from build123d import *

# Parameters (mm, degrees)
SKETCH1_R           = 1.054
BOSS_EXTRUDE1_DEPTH = 3
SKETCH3_R           = 1.1
BOSS_EXTRUDE2_DEPTH = 3
CUT_EXTRUDE1_DEPTH  = 23.736281859
SKETCH4_R           = 1.5
BOSS_EXTRUDE3_DEPTH = 1
FILLET1_R           = 1


with BuildPart() as part:
    # Sketch1 → Boss-Extrude1 (new body)
    with BuildSketch(Plane(origin=(0, 0, 0), x_dir=(1, 0, 0), z_dir=(0, 1, 0))):
        with BuildLine():
            Line((0, 0), (9.035898385, 0))
            ThreePointArc((9.035898385, 0), (10.767949192, 1), (10.767949192, 3))
            Line((10.767949192, 3), (1.732050808, 18.650635095))
            ThreePointArc((1.732050808, 18.650635095), (0, 19.650635095), (-1.732050808, 18.650635095))
            Line((-1.732050808, 18.650635095), (-10.767949192, 3))
            ThreePointArc((-10.767949192, 3), (-10.767949192, 1), (-9.035898385, 0))
            Line((-9.035898385, 0), (0, 0))
        make_face()
        with Locations(Location((0, 17.650635095, 0), (0, 0, 270))):
            Circle(SKETCH1_R, mode=Mode.SUBTRACT)
        with Locations(Location((-9.035898385, 2, 0), (0, 0, 270))):
            Circle(SKETCH1_R, mode=Mode.SUBTRACT)
        with Locations(Location((9.035898385, 2, 0), (0, 0, 270))):
            Circle(SKETCH1_R, mode=Mode.SUBTRACT)
    extrude(amount=BOSS_EXTRUDE1_DEPTH)

    # Sketch3 → Boss-Extrude2 (add)
    with BuildSketch(Plane(origin=(0, 3, 0), x_dir=(1, 0, 0), z_dir=(0, 1, 0))):
        with BuildLine():
            Line((-9.526279442, 14.216878365), (9.526279442, 14.216878365))
            ThreePointArc((9.526279442, 14.216878365), (10.825317547, 13.466878365), (10.825317547, 11.966878365))
            Line((10.825317547, 11.966878365), (1.299038106, -4.533121635))
            ThreePointArc((1.299038106, -4.533121635), (0, -5.283121635), (-1.299038106, -4.533121635))
            Line((-1.299038106, -4.533121635), (-10.825317547, 11.966878365))
            ThreePointArc((-10.825317547, 11.966878365), (-10.825317547, 13.466878365), (-9.526279442, 14.216878365))
        make_face()
        with Locations(Location((0, -3.783121635, 0), (0, 0, 270))):
            Circle(SKETCH3_R, mode=Mode.SUBTRACT)
        with Locations(Location((-9.526279442, 12.716878365, 0), (0, 0, 270))):
            Circle(SKETCH3_R, mode=Mode.SUBTRACT)
        with Locations(Location((9.526279442, 12.716878365, 0), (0, 0, 270))):
            Circle(SKETCH3_R, mode=Mode.SUBTRACT)
    extrude(amount=-BOSS_EXTRUDE2_DEPTH)

    # Sketch2 → Cut-Extrude1 (cut, through all)
    with BuildSketch(Plane(origin=(0, 3, 0), x_dir=(1, 0, 0), z_dir=(0, 1, 0))):
        with BuildLine():
            Line((-1, 15.918584287), (-8.035898385, 3.732050808))
            ThreePointArc((-8.035898385, 3.732050808), (-7.303847577, 3), (-7.035898385, 2))
            Line((-7.035898385, 2), (7.035898385, 2))
            ThreePointArc((7.035898385, 2), (7.303847577, 3), (8.035898385, 3.732050808))
            Line((8.035898385, 3.732050808), (1, 15.918584287))
            ThreePointArc((1, 15.918584287), (0, 15.650635095), (-1, 15.918584287))
        make_face()
    extrude(amount=-CUT_EXTRUDE1_DEPTH, mode=Mode.SUBTRACT)

    # Sketch4 → Boss-Extrude3 (add)
    with BuildSketch(Plane.XZ):
        with Locations(Location((0, 3.783121635, 0), (0, 0, 30))):
            Circle(SKETCH4_R)
        with Locations(Location((9.526279442, -12.716878365, 0), (0, 0, 270))):
            Circle(SKETCH4_R)
        with Locations(Location((-9.526279442, -12.716878365, 0), (0, 0, 270))):
            Circle(SKETCH4_R)
    extrude(amount=BOSS_EXTRUDE3_DEPTH)

    # Fillet1
    fillet1_edges = [part.edges().sort_by_distance(p)[0] for p in [
        (-1.299038106, -1, 3.033121635),
        (9.526279442, -1, -11.216878365),
        (-9.526279442, -1, -11.216878365),
    ]]
    fillet(fillet1_edges, radius=FILLET1_R - 0.0001)  # a hair under: the kernel refuses the full size


solid = part.part
Model file for the job. Use its own axes, mm. A direction names the side the tool comes from. Coordinates: 2 decimals unless noted, no trailing zeros. Order: outer loops, then holes, each group sorted by start corner. A loop starts at its lowest first (then second) coordinate and runs counter-clockwise, first axis right, second up. Notation, with made-up numbers: (69.25, -10.75) -> (76.25, -10.75) arc R16 ccw to (76.25, 13.25) -> close; hole circle Ø2 at (36, -27). An arc over 180 degrees is marked (long way). Return JSON: item names as keys, results as strings. Group by question number.
Item 1: Saw through at A-A on y = 2.2. State how many separate pieces and enclosed holes the cut face has, then the cut area to 3 significant figures.
Item 2: Pull direction X, two halves, no side cores. Call faces 1 (the flat face through (-9.5, 1.52, -9.67)), 2 (the flat face through (0, -1, 4)), 3 (the flat face through (3.03, 1.48, -16.4)), 4 (the cylindrical face through (7.3, 1.52, -2.99)): pulls with the +X half, pulls with the -X half, needs draft (parallel to the pull), parting line crosses it, or undercut.
Item 3: Flat gauge pins, fed straight in: P1, Ø10, axis at x = 5.5, z = -5, coming from the -Y side; P2, Ø1.5, axis at x = 7.5, y = 1.5, coming from the +Z side; P3, Ø0.9, axis at x = -8, y = 1, coming from the -Z side. Where does each tip first touch, or does it go through?
Item 4: Saw through at B-B on x = -3.25. Write the cut outline in (y, z), then the cut area to 3 significant figures.
Item 5: Wall check: line 1 along X through (y, z) = (1.15, -1.75); line 2 along X through (y, z) = (0.75, -12.25); line 3 along Z through (x, y) = (9.25, 2.4). Give the ranges that are in metal, low to high. Write a range as [from, to].
Item 6: Tool access for faces 5 (the flat face through (-9.5, 1.5, -5.2)), 6 (the flat face through (9.5, 1.5, -5.2)), 7 (the flat face through (-10, 0, -13)), 8 (the flat face through (0, 2, -2)): list every direction of +Z, -Z, +X, -X, +Y, -Y with a clear straight run to the whole face (end or side of a thin tool).
Item 7: Saw through at C-C on z = -8.5. Write the cut outline in (x, y).
Values found:
{
 "1": {"separate pieces": "1", "enclosed holes": "7", "area": "180 mm2"},
 "2": {"face 1": "pulls with the -X half", "face 2": "needs draft", "face 3": "pulls with the +X half", "face 4": "undercut"},
 "3": {"P1": "stops at y = 0", "P2": "stops at z = 0", "P3": "stops at z = -14.22"},
 "4": {"outline": "(0, -16.02) -> (3, -16.02) -> (3, -12.02) -> (0, -12.02) -> close; (0, -2) -> (3, -2) -> (3, 1.15) -> (0, 1.15) -> close", "area": "21.5 mm2"},
 "5": {"line 1": "x = [-11.02, -10.06], [-8.01, 8.01], [10.06, 11.02]", "line 2": "x = [-10.95, -10.52], [-8.53, -3.12], [3.12, 8.53], [10.52, 10.95]", "line 3": "z = [-14.22, -13.78], [-11.65, -9.24], [-5.63, -3.03], [-0.97, -0.01]"},
 "6": {"face 5": "-X, +Y, -Y", "face 6": "+X, +Y, -Y", "face 7": "+Y", "face 8": "+Y, -Y"},
 "7": {"outline": "(-8.82, 0) -> (-5.28, 0) -> (-5.28, 3) -> (-8.82, 3) -> close; (5.28, 0) -> (8.82, 0) -> (8.82, 3) -> (5.28, 3) -> close"}
}
